Geometry: final body of the model. Coordinates: model frame, mm. Round coordinates to 2 decimals unless told otherwise and drop trailing zeros. Loops run counter-clockwise (first coordinate to the right, second up) from the corner with the lowest first, then second, coordinate; pieces in that order, holes last. Notation, with made-up numbers: M -33,5 L -29,5 A28 cw -29,31 Z; hole C 20.25,-4 d8. An arc over 180 degrees is marked long. Answer as a JSON object with one key per item and string values.
```python
from build123d import *

# Parameters (mm, degrees)
F1_DEPTH    = 6
F2_R        = 6
F3_SIZE2    = 5.6
F3_SIZE     = 5.64
F4_T1_DEPTH = 6


# Not quite as in the source:
# - a fillet or chamfer that OpenCascade refuses, or shapes differently, is made with other operations: its cross-section is extruded or revolved along the edge and cut away or added


with BuildPart() as f1:
    # F0 (on Front) → F1 (new body)
    with BuildSketch(Plane.XZ):
        with BuildLine():
            Line((-43.5, -10.06), (0, -15.282))
            Line((0, -15.282), (0, 74.41))
            ThreePointArc((0, 74.41), (-7.3393922947, 76.4880320104), (-12.5, 82.1052398935))
            Line((-12.5, 82.1052398935), (-12.5, 8.61))
            Line((-12.5, 8.61), (-50, 8.61))
            Line((-50, 8.61), (-50, 2.11))
            Line((-50, 2.11), (-43.5, 2.11))
            Line((-43.5, 2.11), (-43.5, -10.06))
        make_face()
        with BuildLine():
            ThreePointArc((-12.5, 82.1052398935), (-7.3393922947, 76.4880320104), (0, 74.41))
            Line((0, 74.41), (0, 90.615))
            ThreePointArc((0, 90.615), (-1.4849242405, 91.2300757595), (-2.1, 92.715))
            Line((-2.1, 92.715), (-2.1, 95.715))
            ThreePointArc((-2.1, 95.715), (-1.4849242405, 97.1999242405), (0, 97.815))
            Line((0, 97.815), (0, 102.41))
            ThreePointArc((0, 102.41), (-7.3393922947, 100.3319679896), (-12.5, 94.7147601065))
            Line((-12.5, 94.7147601065), (-12.5, 82.1052398935))
        make_face()
    extrude(amount=-F1_DEPTH)

    # F2
    f2_edges = [f1.edges().sort_by_distance(p)[0] for p in [
        (-43.5, 3, 2.11),
    ]]
    fillet(f2_edges, radius=F2_R)

    # F3
    f3_edges = [f1.edges().sort_by_distance(p)[0] for p in [
        (-21.75, 0, -12.671),
    ]]
    f3_side = f1.faces().sort_by_distance((-42.221274, 0, -6.975))[0]
    chamfer(f3_edges, length=F3_SIZE, length2=F3_SIZE2, reference=f3_side)

    # F4: fillet of radius 100 on 1 edges, made by hand

    # F4_s2 → F4_t1 (join)
    with BuildSketch(Plane.XZ.offset(-6)):
        with BuildLine():
            ThreePointArc((-50, 8.61), (-22.3612181134, 43.3712047908), (-12.5, 86.67247498))
            Line((-12.5, 86.67247498), (-12.5, 8.61))
            Line((-12.5, 8.61), (-50, 8.61))
        make_face()
    extrude(amount=F4_T1_DEPTH)

    # F5: F1 across plane


with BuildPart() as f1_1:
    add(f1.part)
    add(f1.part.mirror(Plane.YZ))


solid = f1_1.part
```
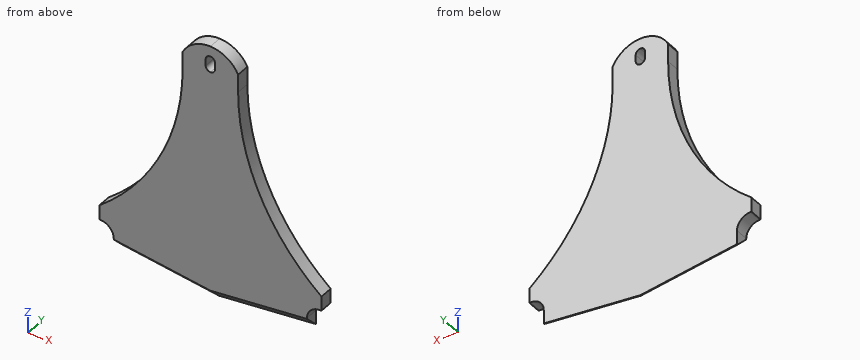
1) First-contact query: pin 1 (3 mm diameter, centred on y = 2, z = -8.5, fed in from +X); pin 2 (0.6 mm diameter, centred on x = 49.5, y = 2, fed in from -Z); pin 3 (1.5 mm diameter, centred on y = 3, z = 12, fed in from +X). Flat tips, straight axial feed; report the tip coordinate or a pass-through.
Geometry results:
{"pin 1": "x = 43.5", "pin 2": "z = 2.1", "pin 3": "x = 46.84"}
2) Cut plane D-D on x = -29.5. Return the cut outline in (y, z).
Geometry results:
{"outline": "M 0,-6.06 L 5.6,-11.74 L 6,-11.74 L 6,30.9 L 0,30.9 Z"}
3) Cut plane B-B on x = 5. Return the cut outline in (y, z).
Geometry results:
{"outline": "M 0,-9 L 5.6,-14.68 L 6,-14.68 L 6,101.49 L 0,101.49 Z"}
4) Cut plane A-A on y = 4.5. Return the cut outline in (x, z) (3 decimals).
Geometry results:
{"outline": "M -50,2.11 L -49.5,2.11 A6 cw -43.5,-3.89 L -43.5,-8.944 L 0,-14.166 L 43.5,-8.944 L 43.5,-3.89 A6 cw 49.5,2.11 L 50,2.11 L 50,8.61 A100 cw 12.5,86.672 L 12.5,94.715 A14 ccw -12.5,94.715 L -12.5,86.672 A100 cw -50,8.61 Z; hole M -2.1,92.715 A2.1 ccw 2.1,92.715 L 2.1,95.715 A2.1 ccw -2.1,95.715 Z"}
5) Cut plane C-C on z = 32.5. Return the cut outline in (x, y).
Geometry results:
{"outline": "M -28.44,0 L 28.44,0 L 28.44,6 L -28.44,6 Z"}
6) Line query: probe 1 along X at (y, z) = (0.5, 96.5); probe 2 along Z at (x, y) = (5, 4.75); probe 3 along X at (y, z) = (2.5, 49.5). Output: solid intervals per line, ascending.
Geometry results:
{"probe 1": "-11.43 to -1.95, 1.95 to 11.43", "probe 2": "-13.82 to 101.49", "probe 3": "-19.67 to 19.67"}
